Geometry: final body of the model. Coordinates: model frame, mm. A direction names the side the tool comes from. Give positions to 0.01 mm unless a question says otherwise; leave off trailing zeros. Order: outer loops, then holes, each group sorted by start corner. A loop starts at its lowest first (then second) coordinate and runs counter-clockwise, first axis right, second up. Notation, with made-up numbers: (55.5, 89.5) -> (88.5, 89.5) arc R25 ccw to (88.5, 106.5) -> close; hole circle Ø7 at (69.25, -3). An arc over 180 degrees is marked (long way). Answer in a Markdown table with one row per item. Add a question column.
Q1. Contact query for flat-ended pins moving along their axis: P1, Ø3, axis at x = 15, z = 15, coming from the +Y side; P2, Ø0.7, axis at x = -15, z = -15, coming from the +Y side; P3, Ø2.5, axis at y = 48.5, z = -0.5, coming from the -X side. Output: stop coordinate, or through.
Q2. Line query: line 1 along Z through (x, y) = (-15, 33); line 2 along X through (y, z) = (38.4, 0). Output: solid intervals per line, ascending. Write a range as from..to.
Q3. Cut plane A-A on y = 33. Return the cut outline in (x, z).
Q4. Cut plane D-D on y = 13.5. Return the cut outline in (x, z).
Q5. Cut plane C-C on z = -15. Return the cut outline in (x, y), and give its area (3 significant figures).
Q6. Pull-direction query (Z, two-part tool) for faces 1 (the face through (0, 48, 1.5)), 2 (the face through (24, 6, -8.5)), 3 (the face through (-1.5, 48, 0)), 4 (the face through (13.963, 33.038, 15.661)); classes: +Z half, -Z half, draft (parallel to the pull), parting line (faces both ways), or undercut.
Q7. Set-up query: faces 5 (the face through (0, 18, -21)), 6 (the face through (-2.17, 38.49, -9.76)), 7 (the face through (1.5, 48, 0)), 8 (the face through (24, 6, 8.5)), 9 (the face through (0, 48, -1.5)). Return all of +Z, -Z, +X, -X, +Y, -Y with unobstructed straight access to the full face (end or side cutting, diameter ignored); none if empty.
Q8. Cut plane B-B on x = 0. Return the cut outline in (y, z).
Autodesk Inventor part; units mm, degrees
ref_plane "YZ Plane" through (0, 0, 0) normal (1, 0, 0) x (0, 1, 0)
ref_plane "XZ Plane" through (0, 0, 0) normal (0, 1, 0) x (-1, 0, 0)
ref_plane "XY Plane" through (0, 0, 0) normal (0, 0, 1) x (1, 0, 0)
sketch "Sketch1" plane through (0, 0, 0) normal (0, 1, 0) x (-1, 0, 0)
  line L0 (21, 21) -> (-21, 21)
  line L1 (-21, 21) -> (-21, -21)
  line L2 (-21, -21) -> (21, -21)
  line L3 (21, -21) -> (21, 21)
  line L4 (21, 21) -> (-21, -21) construction
  line L5 (-21, 21) -> (21, -21) construction
  point P0 (0, 0)
  dimension "d0" = 42
  dimension "d1" = 42
extrude "Extrusion1" add sketch "Sketch1" along normal blind 37.5
fillet "Fillet1" radius 5 4 edges at (21, 18.75, 21) (21, 18.75, -21) (-21, 18.75, -21) (-21, 18.75, 21)
sketch "Sketch2" plane through (0, 37.5, 0) normal (0, 1, 0) x (1, 0, 0)
  arc A0 (-21, -16) -> (-16, -21) centre (-16, -16) ccw
  line L0 (-16, -21) -> (16, -21)
  arc A1 (16, -21) -> (21, -16) centre (16, -16) ccw
  line L1 (21, -16) -> (21, 16)
  arc A2 (21, 16) -> (16, 21) centre (16, 16) ccw
  line L2 (16, 21) -> (-16, 21)
  arc A3 (-16, 21) -> (-21, 16) centre (-16, 16) ccw
  line L3 (-21, 16) -> (-21, -16)
  circle A4 centre (0, 0) radius 11
  circle A5 centre (0, 0) radius 10
  point P0 (-15, -15)
  point P1 (15, -15)
  point P2 (15, 15)
  point P3 (-15, 15)
  dimension "d5" = 22
  dimension "d6" = 20
  dimension "d7" = 6
  dimension "d8" = 6
  dimension "d11" = 360
extrude "Extrusion2" add sketch "Sketch2" along normal blind 2 contours A4
hole "Hole1" at (-15, 37.5, 15) at (15, 37.5, 15) at (15, 37.5, -15) at (-15, 37.5, -15) direction (0, -1, 0) diameter 2.459 depth 8.8
sketch "Sketch3" plane through (0, 37.5, 0) normal (0, 1, 0) x (1, 0, 0)
  circle A0 centre (0, 0) radius 2.5
  dimension "d22" = 5
extrude "Extrusion3" add sketch "Sketch3" along normal blind 6
chamfer "Chamfer1" distance 0.5 angle 45 1 edges at (-2.5, 43.5, 0)
sketch "Sketch4" plane through (0, 43.5, 0) normal (0, 1, 0) x (1, 0, 0)
  line L0 (-1.5, 1.5) -> (1.5, 1.5)
  line L1 (1.5, 1.5) -> (1.5, -1.5)
  line L2 (1.5, -1.5) -> (-1.5, -1.5)
  line L3 (-1.5, -1.5) -> (-1.5, 1.5)
  line L4 (-1.5, 1.5) -> (1.5, -1.5) construction
  line L5 (1.5, 1.5) -> (-1.5, -1.5) construction
  point P0 (0, 0)
  dimension "d28" = 3
  dimension "d29" = 3
extrude "Extrusion4" add sketch "Sketch4" along normal blind 8.6
sketch "Sketch5" plane through (21, 0, 16) normal (1, 0, 0) x (0, 0, -1)
  line L0 (7.5, 12) -> (24.5, 12)
  line L1 (24.5, 12) -> (24.5, 0)
  line L2 (24.5, 0) -> (7.5, 0)
  line L3 (7.5, 0) -> (7.5, 12)
  line L4 (7.5, 12) -> (24.5, 0) construction
  line L5 (24.5, 12) -> (7.5, 0) construction
  line L6 (0, 0) -> (32, 0)
  point P0 (16, 0)
  point P1 (16, 6)
  point P2 (16, 0)
  dimension "d32" = 17
  dimension "d33" = 12
extrude "Extrusion5" add sketch "Sketch5" along normal blind 6
properties part number "steppeSquare"
Completed:
| question | item | result |
|---|---|---|
| 1 | P1 | stops at y = 37.5 |
| 1 | P2 | stops at y = 28.7 |
| 1 | P3 | stops at x = -1.5 |
| 2 | line 1 | z = -21..-16.23, -13.77..13.77, 16.23..21 |
| 2 | line 2 | x = -11..-10, -2.5..2.5, 10..11 |
| 3 | outline | (-21, -16) arc R5 ccw to (-16, -21) -> (16, -21) arc R5 ccw to (21, -16) -> (21, 16) arc R5 ccw to (16, 21) -> (-16, 21) arc R5 ccw to (-21, 16) -> close; hole circle Ø2.46 at (-15, -15); hole circle Ø2.46 at (-15, 15); hole circle Ø2.46 at (15, -15); hole circle Ø2.46 at (15, 15) |
| 4 | outline | (-21, -16) arc R5 ccw to (-16, -21) -> (16, -21) arc R5 ccw to (21, -16) -> (21, 16) arc R5 ccw to (16, 21) -> (-16, 21) arc R5 ccw to (-21, 16) -> close |
| 5 | outline | (-21, 0) -> (21, 0) -> (21, 37.5) -> (16.23, 37.5) -> (16.23, 28.7) -> (13.77, 28.7) -> (13.77, 37.5) -> (-13.77, 37.5) -> (-13.77, 28.7) -> (-16.23, 28.7) -> (-16.23, 37.5) -> (-21, 37.5) -> close |
| 5 | area | 1,530 mm² |
| 6 | face 1 | +Z half |
| 6 | face 2 | -Z half |
| 6 | face 3 | draft |
| 6 | face 4 | undercut |
| 7 | face 5 | -Z, +X, -X, +Y, -Y |
| 7 | face 6 | +Y |
| 7 | face 7 | +Z, -Z, +X, +Y |
| 7 | face 8 | +Z, +X, +Y, -Y |
| 7 | face 9 | -Z, +X, -X, +Y |
| 8 | outline | (0, -21) -> (37.5, -21) -> (37.5, -11) -> (39.5, -11) -> (39.5, -10) -> (37.5, -10) -> (37.5, -2.5) -> (43, -2.5) -> (43.5, -2) -> (43.5, -1.5) -> (52.1, -1.5) -> (52.1, 1.5) -> (43.5, 1.5) -> (43.5, 2) -> (43, 2.5) -> (37.5, 2.5) -> (37.5, 10) -> (39.5, 10) -> (39.5, 11) -> (37.5, 11) -> (37.5, 21) -> (0, 21) -> close |
